Geometry: final body of the model. Coordinates: model frame, mm. A direction names the side the tool comes from. Round coordinates to 2 decimals unless told otherwise and drop trailing zeros. Loops run counter-clockwise (first coordinate to the right, second up) from the corner with the lowest first, then second, coordinate; pieces in that order, holes last. Notation, with made-up numbers: (-2, -32.5) -> (8, -32.5) arc R14 ccw to (8, -14.5) -> close; hole circle Ø9 at (1, 66.25). An arc over 180 degrees is marked (long way). Answer in a Markdown table with one row per item.
Autodesk Fusion 360 part; units mm, degrees
sketch "Base Profile" plane through (0, 0, 0) normal (1, 0, 0) x (0, 1, 0)
  line L0 (0, 0) -> (42, 0)
  line L1 (42, 0) -> (42, 42)
  line L2 (42, 42) -> (0, 60)
  line L3 (0, 60) -> (0, 0)
  line L4 (0, 30) -> (42, 12)
  dimension "d1" = 42
  dimension "d2" = 60
  dimension "d3" = 42
  dimension "d4" = 30
extrude "Extrude1" add sketch "Base Profile" against normal blind 16
extrude "Extrude2" add sketch "Base Profile" along normal blind 10 contours L0 L1 L3 L4
sketch "Hole Layouts" plane through (0, 0, 0) normal (0, 0, 1) x (1, 0, 0)
  line L0 (0, 42) -> (0, 0)
  line L1 (0, 0) -> (10, 0)
  line L2 (10, 0) -> (10, 42)
  line L3 (10, 42) -> (0, 42)
  line L4 (0, 0) -> (0, 42)
  line L5 (0, 42) -> (-16, 42)
  line L6 (-16, 42) -> (-16, 0)
  line L7 (-16, 0) -> (0, 0)
  circle A0 centre (-8, 7.65) radius 4.65
  circle A1 centre (-8, 18.45) radius 4.15
  circle A2 centre (-8, 28.25) radius 3.65
  circle A3 centre (-8, 36.8) radius 2.9
  line L8 (5, 0) -> (5, 42) construction
  circle A4 centre (5, 5.65) radius 2.65
  circle A5 centre (5, 14.4) radius 2.4
  circle A6 centre (5, 22.65) radius 2.15
  circle A7 centre (5, 30.4) radius 1.9
  circle A8 centre (5, 37.65) radius 1.65
  line L9 (-8, 0) -> (-8, 42) construction
  dimension "d10" = 9.3
  dimension "d11" = 8.3
  dimension "d12" = 7.3
  dimension "d13" = 5.8
  dimension "d15" = 2
  dimension "d16" = 2
  dimension "d17" = 2
  dimension "d19" = 3
  dimension "d20" = 2.3
  dimension "d21" = 5.3
  dimension "d22" = 4.8
  dimension "d23" = 4.3
  dimension "d24" = 3.8
  dimension "d25" = 3.3
  dimension "d26" = 3.7
  dimension "d27" = 3.7
  dimension "d29" = 3.7
  dimension "d30" = 3.7
  dimension "d32" = 2.7
  dimension "d33" = 3
extrude "Extrude3" cut sketch "Hole Layouts" along normal through all contours A0 | A1 | A2 | A3 | A4 | A5 | A6 | A7 | A8
fillet "Fillet1" radius 2 5 edges at (0, 42, 27) (10, 42, 6) (10, 0, 15) (-16, 42, 21) (-16, 0, 30)
sketch "Clipping corners for Printing" plane through (-16, 0, 0) normal (-1, 0, 0) x (0, -1, 0)
  line L0 (-2, 0) -> (-2, 59.1429)
  line L1 (-2, 59.1429) -> (-40, 42.8571)
  line L2 (-40, 42.8571) -> (-40, 0)
  line L3 (-40, 0) -> (-2, 0)
  line L4 (-42, 42) -> (0, 60)
  line L5 (0, 60) -> (0, 0)
  line L6 (-2, 59.1429) -> (0, 59.1429)
  line L7 (-2, 59.1429) -> (-40, 42.8571)
  line L8 (0, 30) -> (-42, 12)
  line L9 (-2, 0) -> (-2, 29.1429)
  line L10 (-2, 29.1429) -> (0, 29.1429)
  point P0 (-3, 58.7143)
extrude "Extrude4" cut sketch "Clipping corners for Printing" against normal through all contours L4 L5 L6
extrude "Extrude5" cut sketch "Clipping corners for Printing" along normal up to surface (10 mm away) from surface at -26 contours L5 L8 L10
fillet "Fillet2" radius 2 1 edges at (0, 0, 44.1429)
equation "d10 = 9 mm + SlipFitTolerance"
equation "d11 = 8 mm + SlipFitTolerance"
equation "d12 = 7 mm + SlipFitTolerance"
equation "d13 = 5.5 mm + SlipFitTolerance"
equation "d16 = d15"
equation "d17 = d15"
equation "d21 = 5 mm + SlipFitTolerance"
equation "d22 = 4.5 mm + SlipFitTolerance"
equation "d23 = 4 mm + SlipFitTolerance"
equation "d24 = 3.5 mm + SlipFitTolerance"
equation "d25 = 3 mm + SlipFitTolerance"
equation "d27 = d26"
equation "d29 = d26"
equation "d30 = d26"
equation "SlipFitTolerance = 0.3 mm"
Item 1: Ray query, L1, parallel to Y at x = -8, z = 22.5; L2, parallel to Y at x = 5, z = 5.5; L3, parallel to X at y = 22.65, z = 13.75. Return the intervals inside material, ascending.
Ans:
| item | result |
|---|---|
| L1 | 0 to 3, 12.3 to 14.3, 22.6 to 24.6, 31.9 to 33.9, 39.7 to 42 |
| L2 | 0 to 3, 8.3 to 12, 16.8 to 20.5, 24.8 to 28.5, 32.3 to 36, 39.3 to 42 |
| L3 | -16 to 2.85, 7.15 to 10 |
Item 2: Section query B-B, the plane y = 25.5. Output: boundary loops of the cut face in (x, z).
Ans:
| item | result |
|---|---|
| outline | (-16, 0) -> (-10.4, 0) -> (-10.4, 49.07) -> (-16, 49.07) -> close; (-5.6, 0) -> (10, 0) -> (10, 19.07) -> (0, 19.07) -> (0, 49.07) -> (-5.6, 49.07) -> close |
Item 3: Section query C-C, the plane x = 5. Output: boundary loops of the cut face in (y, z).
Ans:
| item | result |
|---|---|
| outline | (0, 0) -> (3, 0) -> (3, 28.71) -> (2, 29.14) -> (0, 29.14) -> close; (8.3, 0) -> (12, 0) -> (12, 24.86) -> (8.3, 26.44) -> close; (16.8, 0) -> (20.5, 0) -> (20.5, 21.21) -> (16.8, 22.8) -> close; (24.8, 0) -> (28.5, 0) -> (28.5, 17.79) -> (24.8, 19.37) -> close; (32.3, 0) -> (36, 0) -> (36, 14.57) -> (32.3, 16.16) -> close; (39.3, 0) -> (42, 0) -> (42, 12) -> (39.3, 13.16) -> close |
Item 4: Section query A-A, the plane z = 31.5. Output: boundary loops of the cut face in (x, y), and give its area (3 significant figures).
Ans:
| item | result |
|---|---|
| outline | (-16, 2) arc R2 ccw to (-14, 0) -> (-2, 0) arc R2 ccw to (0, 2) -> (0, 40) arc R2 ccw to (-2, 42) -> (-14, 42) arc R2 ccw to (-16, 40) -> close; hole circle Ø9.3 at (-8, 7.65); hole circle Ø8.3 at (-8, 18.45); hole circle Ø7.3 at (-8, 28.25); hole circle Ø5.8 at (-8, 36.8) |
| area | 478 mm2 |
Item 5: Section query D-D, the plane y = 7.65. Output: boundary loops of the cut face in (x, z).
Ans:
| item | result |
|---|---|
| outline | (-16, 0) -> (-12.65, 0) -> (-12.65, 56.72) -> (-16, 56.72) -> close; (-3.35, 0) -> (3.26, 0) -> (3.26, 26.72) -> (0, 26.72) -> (0, 56.72) -> (-3.35, 56.72) -> close; (6.74, 0) -> (10, 0) -> (10, 26.72) -> (6.74, 26.72) -> close |
Item 6: Set-up query: faces 4 (the cylindrical face through (-0.6, 0.57, 44.35)), 5 (the cylindrical face through (-0.57, 41.4, 27.64)), 6 (the flat face through (-6, 42, 16)). Return all of +Z, -Z, +X, -X, +Y, -Y with unobstructed straight access to the full face (end or side cutting, diameter ignored); none if empty.
Ans:
| item | result |
|---|---|
| face 4 | +Z, +X, -Y |
| face 5 | +Z, +X, +Y |
| face 6 | +Z, -Z, +X, -X, +Y |
Item 7: Mould query, pull axis Y, two halves, no side actions, for faces 1 (the cylindrical face through (-8.54, 14.335, 26.562)), 2 (the flat face through (10, 17, 12)), 3 (the flat face through (-6, 0, 23)). Classes: released by +Y, released by -Y, zero draft, split by the parting line, or undercut.
Ans:
| item | result |
|---|---|
| face 1 | undercut |
| face 2 | zero draft |
| face 3 | released by -Y |
Item 8: First-contact query: P1, Ø1.5, axis at x = -1.5, y = 12.5, coming from the +Z side; P2, Ø4, axis at x = -2.5, z = 45.5, coming from the +Y side; P3, Ø1, axis at x = -3.5, y = 27.5, coming from the +Z side. Flat tips, straight axial feed; report the tip coordinate or a pass-through.
Ans:
| item | result |
|---|---|
| P1 | z = 54.96 |
| P2 | y = 38.5 |
| P3 | z = 48.43 |
